Here's the drawing with two shaded views (mm, measured from the low corner). I have some questions. Give positions to 0.01 mm unless a question says otherwise; leave off trailing zeros. Write each loop counter-clockwise with the first axis right and the second up, starting at its lowest first coordinate (ties: lowest second). Pieces come first, ordered by that corner, then holes.
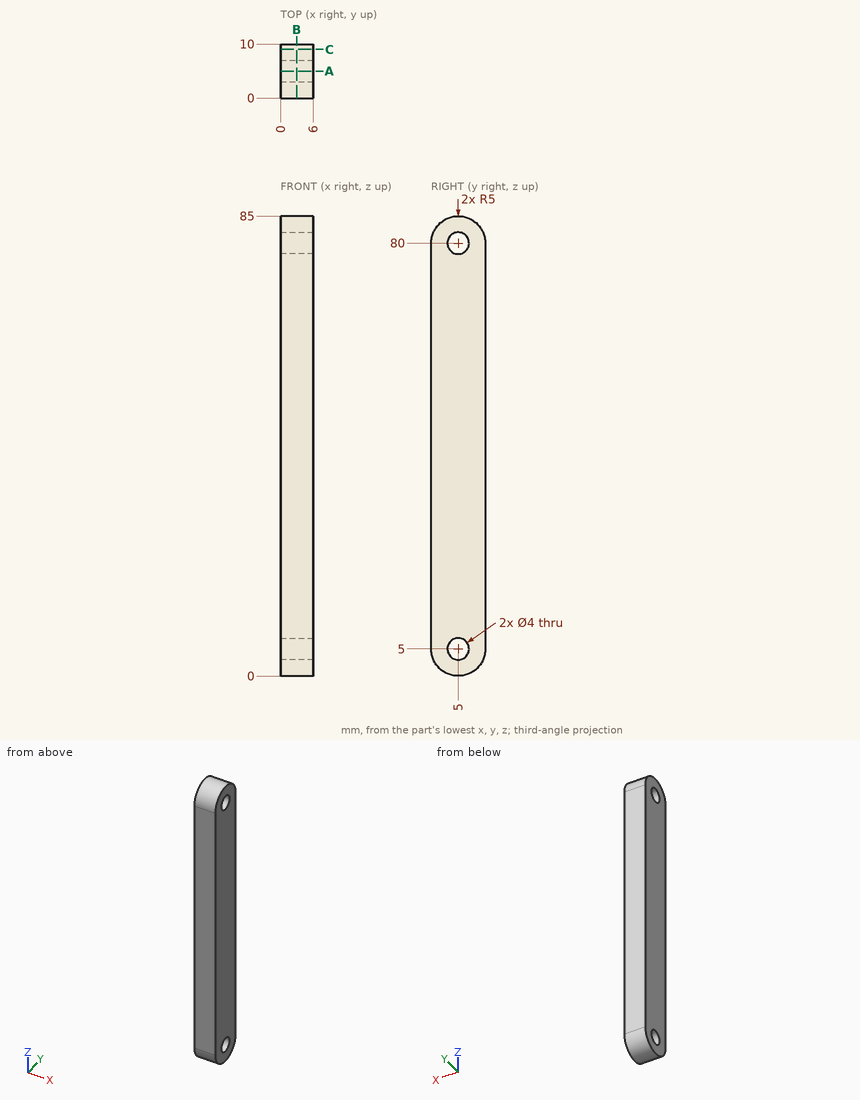
(1) Imagine slicing it at B-B, the plane x = 2.95. Write out the boundary of the cut face in (y, z).
Returned:
outline: (0, 5) arc R5 ccw to (10, 5) - (10, 80) arc R5 ccw to (0, 80) - close; hole circle Ø4 at (5, 5); hole circle Ø4 at (5, 80)
(2) Will this pin go through, and if not, where does the flat tip stop? P1, Ø2, axis at x = 1, z = 28.5, coming from the -Y side.
Returned:
P1: stops at y = 0
(3) Imagine slicing it at A-A, the plane y = 5. Write out the boundary of the cut face in (x, z), plus the area to 3 significant figures.
Returned:
outline: (0, 0) - (6, 0) - (6, 3) - (0, 3) - close; (0, 7) - (6, 7) - (6, 78) - (0, 78) - close; (0, 82) - (6, 82) - (6, 85) - (0, 85) - close
area: 462 mm2
(4) Imagine slicing it at C-C, the plane y = 9. Write out the boundary of the cut face in (x, z).
Returned:
outline: (0, 2) - (6, 2) - (6, 83) - (0, 83) - close
(5) If I drill on L1, parallel to Z at x = 1.3, y = 4.75; L2, parallel to Z at x = 1.15, y = 6; L3, parallel to Y at x = 3.05, z = 5, over which ranges is the centre line in solid material (lowest first)?
Returned:
L1: z = 0.01 to 3.02, 6.98 to 78.02, 81.98 to 84.99
L2: z = 0.1 to 3.27, 6.73 to 78.27, 81.73 to 84.9
L3: y = 0 to 3, 7 to 10
